Answer from the drawing. Dimensions are ordinates in mm from the lowest x, y and z of the part. A direction names the side the tool comes from. Give positions to 0.01 mm unless a question says otherwise; leave off trailing zeros. Write each loop counter-clockwise with the first axis right and the second up, starting at its lowest first coordinate (ties: lowest second). Pieces come first, ordered by that corner, then holes.
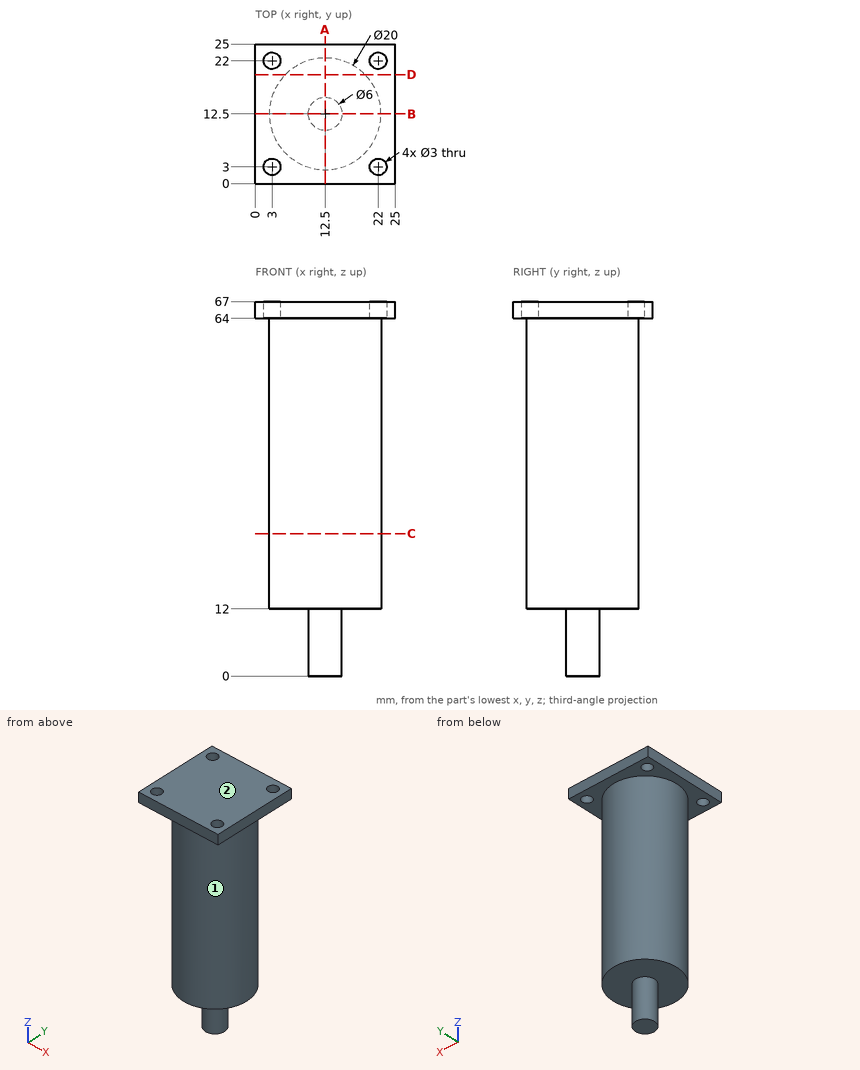
Item 1: A cutting plane is placed at A-A, the plane x = 12.5. Give the vertices of the cut face in (y, z), plus the area to 3 significant figures.
Conclusion:
outline: (0, 64) - (2.5, 64) - (2.5, 12) - (9.5, 12) - (9.5, 0) - (15.5, 0) - (15.5, 12) - (22.5, 12) - (22.5, 64) - (25, 64) - (25, 67) - (0, 67) - close
area: 1,190 mm2
Item 2: A cutting plane is placed at C-C, the plane z = 25.5. Give the vertices of the cut face in (x, y).
Conclusion:
outline: circle Ø20 at (12.5, 12.5)
Item 3: Each of these flat-tipped pins is pushed along its axis until it touches: P1, Ø2, axis at x = 13.5, z = 34.5, coming from the -Y side; P2, Ø8, axis at x = 18.5, y = 7.5, coming from the -Z side; P3, Ø2, axis at y = 13.5, z = 11.5, coming from the +X side; P4, Ø2.5, axis at x = 3, y = 22, coming from the +Z side. Where does it stop, or does it pass through?
Conclusion:
P1: stops at y = 2.5
P2: stops at z = 12
P3: stops at x = 22.5
P4: passes through
Item 4: Consider probe 1 along Y at (x, z) = (3, 65.2); probe 2 along Z at (x, y) = (15.75, 2.75); probe 3 along Z at (x, y) = (8, 17.75). Determine where each line is inside the solid, lowest interval first.
Conclusion:
probe 1: y = 0 to 1.5, 4.5 to 20.5, 23.5 to 25
probe 2: z = 64 to 67
probe 3: z = 12 to 67
Item 5: A cutting plane is placed at D-D, the plane y = 19.5. Give the vertices of the cut face in (x, z).
Conclusion:
outline: (0, 64) - (5.36, 64) - (5.36, 12) - (19.64, 12) - (19.64, 64) - (25, 64) - (25, 67) - (0, 67) - close
Item 6: Which of the six approach directions +Z, -Z, +X, -X, +Y, -Y give full straight-line access (tool end or side, diameter ignored) to the marked faces 1 and 2?
Conclusion:
face 1: -Z
face 2: +Z, +X, -X, +Y, -Y
